```python
from build123d import *

# Parameters (mm, degrees)
SKETCH1_R           = 15.875
SKETCH1_R_2         = 1.75
SKETCH1_R_3         = 1.25
BOSS_EXTRUDE1_DEPTH = 2.54
BOSS_EXTRUDE2_START = -7.110000004
SKETCH1_3_R         = 3.175
SKETCH1_3_R_2       = 1.75
BOSS_EXTRUDE2_DEPTH = 7.110000004


with BuildPart() as part:
    # Sketch1 → Boss-Extrude1 (new body)
    with BuildSketch(Plane.XY):
        Circle(SKETCH1_R)
        with Locations((0, 12.7)):
            Circle(SKETCH1_R_2, mode=Mode.SUBTRACT)
        with Locations((0, -12.7)):
            Circle(SKETCH1_R_2, mode=Mode.SUBTRACT)
        with Locations((-10.16, 6.35)):
            Circle(SKETCH1_R_3, mode=Mode.SUBTRACT)
        with Locations((10.16, 6.35)):
            Circle(SKETCH1_R_3, mode=Mode.SUBTRACT)
        with Locations((10.16, -6.35)):
            Circle(SKETCH1_R_3, mode=Mode.SUBTRACT)
        with Locations((-10.16, -6.35)):
            Circle(SKETCH1_R_3, mode=Mode.SUBTRACT)
    extrude(amount=BOSS_EXTRUDE1_DEPTH)

    # Sketch1<3> → Boss-Extrude2 (add)
    # profile 1 of 2: a face of its own
    with BuildSketch(Plane.XY.offset(BOSS_EXTRUDE2_START)):
        with Locations((0, 12.7)):
            Circle(SKETCH1_3_R)
        with Locations((0, 12.7)):
            Circle(SKETCH1_3_R_2, mode=Mode.SUBTRACT)
    # profile 2 of 2: a face of its own
    with BuildSketch(Plane.XY.offset(BOSS_EXTRUDE2_START)):
        with Locations((0, -12.7)):
            Circle(SKETCH1_3_R)
        with Locations((0, -12.7)):
            Circle(SKETCH1_3_R_2, mode=Mode.SUBTRACT)
    extrude(amount=BOSS_EXTRUDE2_DEPTH)


solid = part.part
```
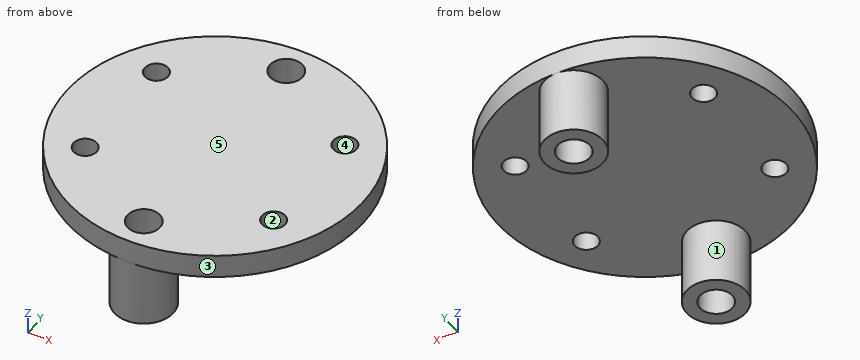
Model file for the job. Use its own axes, mm. Face numbers are marked on the shaded views. A direction names the side the tool comes from. Give positions to 0.01 mm unless a question says otherwise; leave off trailing zeros. Write each loop counter-clockwise with the first axis right and the second up, starting at its lowest first coordinate (ties: lowest second). Pieces come first, ordered by that corner, then holes. Notation, with made-up numbers: M 81,-39 L 120,-39 A21 ccw 120,-9 Z; hole C 26,83.25 d4. An arc over 180 degrees is marked long. Use a Markdown table: item, result.
1) Cut at C-C (z = 0.5). List the corners of the cut face in (x, y) (3 decimals).
Responses:
| item | result |
|---|---|
| outline | C 0,0 d31.75; hole C -10.16,-6.35 d2.5; hole C -10.16,6.35 d2.5; hole C 0,-12.7 d3.5; hole C 0,12.7 d3.5; hole C 10.16,-6.35 d2.5; hole C 10.16,6.35 d2.5 |
2) Cut at B-B (z = -5.25). List the corners of the cut face in (x, y) (3 decimals).
Responses:
| item | result |
|---|---|
| outline | C 0,-12.7 d6.35; C 0,12.7 d6.35; hole C 0,-12.7 d3.5; hole C 0,12.7 d3.5 |
3) Pin check, flat tips, straight feed: pin 1 (1 mm diameter, centred on y = -11.5, z = -1.5, fed in from -X); pin 2 (1 mm diameter, centred on y = 10.5, z = -3.5, fed in from -X); pin 3 (1 mm diameter, centred on y = 11, z = -2.5, fed in from -X); pin 4 (1.5 mm diameter, centred on x = 10.16, y = 6.35, fed in from +Z). Stop position of each tip, or through.
Responses:
| item | result |
|---|---|
| pin 1 | stops at x = -3.1 |
| pin 2 | stops at x = -2.68 |
| pin 3 | stops at x = -2.94 |
| pin 4 | passes through |
4) Drill centre lines: line 1 (Y direction, x = 0, z = 0.75) (3 decimals); line 2 (Y direction, x = 0, z = -0.75) (3 decimals); line 3 (Y direction, x = 10, z = 1.25). Where is each one in solid material? Low to high. Write a range as from..to.
Responses:
| item | result |
|---|---|
| line 1 | y = -15.875..-14.45, -10.95..10.95, 14.45..15.875 |
| line 2 | y = -15.875..-14.45, -10.95..-9.525, 9.525..10.95, 14.45..15.875 |
| line 3 | y = -12.33..-7.59, -5.11..5.11, 7.59..12.33 |
5) Tool access for the marked faces 1 and 2: list every direction of +Z, -Z, +X, -X, +Y, -Y with a clear straight run to the whole face (end or side of a thin tool).
Responses:
| item | result |
|---|---|
| face 1 | -Z |
| face 2 | +Z, -Z |
6) Cut at A-A (y = 12.7). List the corners of the cut face in (x, z) (3 decimals), and give its area (3 significant figures).
Responses:
| item | result |
|---|---|
| outline | M -9.525,0 L -3.175,0 L -3.175,-7.11 L -1.75,-7.11 L -1.75,2.54 L -9.525,2.54 Z; M 1.75,-7.11 L 3.175,-7.11 L 3.175,0 L 9.525,0 L 9.525,2.54 L 1.75,2.54 Z |
| area | 59.8 mm2 |
7) Cut at D-D (x = 10.16). List the corners of the cut face in (y, z).
Responses:
| item | result |
|---|---|
| outline | M -12.2,0 L -7.6,0 L -7.6,2.54 L -12.2,2.54 Z; M -5.1,0 L 5.1,0 L 5.1,2.54 L -5.1,2.54 Z; M 7.6,0 L 12.2,0 L 12.2,2.54 L 7.6,2.54 Z |
8) Pull direction Y, two halves, no side cores. Call the marked faces 3, 4 and 5: +Y half, -Y half, draft (parallel to the pull), parting line (faces both ways), or undercut.
Responses:
| item | result |
|---|---|
| face 3 | parting line |
| face 4 | undercut |
| face 5 | draft |
